For this review, use the dimensioned drawing (mm, ordinates from the lowest corner) and the shaded views. Give positions to 0.01 mm unless a question says otherwise; leave off trailing zeros. Loops run counter-clockwise (first coordinate to the right, second up) from the corner with the lowest first, then second, coordinate; pieces in that order, holes last. Notation, with made-up numbers: M -37,-28.5 L 9,-28.5 A20 cw 9,-0.5 Z; hole C -30.5,70 d7. An arc over 180 degrees is marked long. Use CSV: the item, a comma, the result in double quotes. Start each with the question number.
1. To check wall thickness, follow line 1 (X direction, y = 85, z = 17.25); line 2 (X direction, y = 38, z = 6); line 3 (Y direction, x = 829, z = 6.25). State the ranges of each line that lie inside material, in increasing order. Write a range as [from, to].
2. Take a section at C-C, the plane x = 483. Write out the cut boundary in (y, z).
3. Insertion check: P1, Ø11.5, axis at x = 143.7, y = 38.1, coming from the +Z side; P2, Ø5.5, axis at y = 82.5, z = 9, coming from the -X side; P3, Ø5.5, axis at y = 84.5, z = 9, coming from the +X side; P4, Ø9.5, axis at x = 312, z = 14, coming from the +Y side. Each pin has a flat end and moves straight along its axis. Give the tip position at first contact, or say it passes through.
4. Take a section at A-A, the plane y = 38.1. Write out the cut boundary in (x, z), and give its area (4 significant figures).
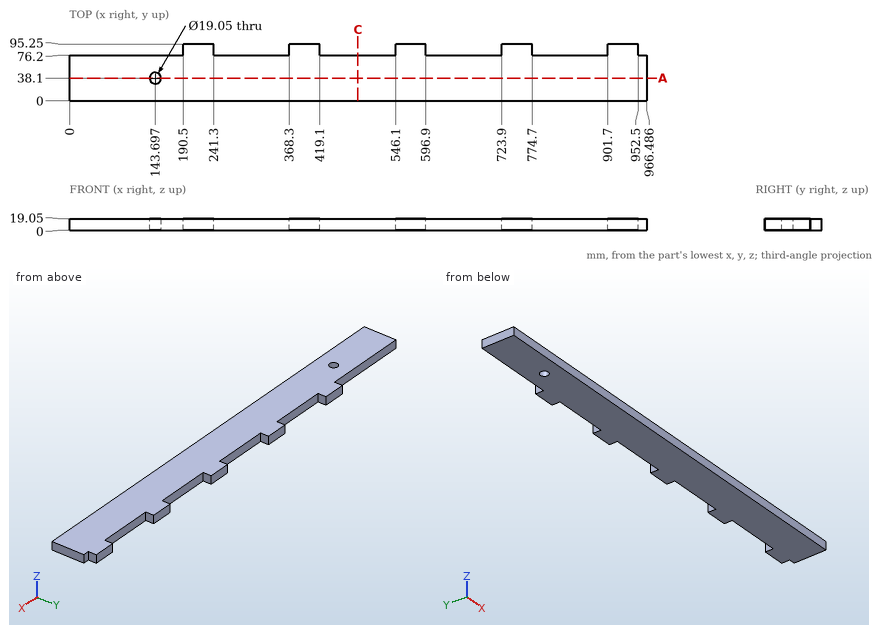
Result set:
1,line 1,"[190.5, 241.3], [368.3, 419.1], [546.1, 596.9], [723.9, 774.7], [901.7, 952.5]"
1,line 2,"[0, 134.17], [153.22, 966.49]"
1,line 3,"[0, 76.2]"
2,outline,"M 0,0 L 76.2,0 L 76.2,19.05 L 0,19.05 Z"
3,P1,"through"
3,P2,"x = 190.5"
3,P3,"x = 952.5"
3,P4,"y = 76.2"
4,outline,"M 0,0 L 134.17,0 L 134.17,19.05 L 0,19.05 Z; M 153.22,0 L 966.49,0 L 966.49,19.05 L 153.22,19.05 Z"
4,area,"18,050 mm2"
